The listing builds one solid part. Answer for the finished solid, in the listing's coordinates (mm). A direction names the side the tool comes from. Round coordinates to 2 decimals unless told otherwise and drop trailing zeros. Write each loop counter-clockwise with the first axis right and the second up, starting at its lowest first coordinate (ties: lowest second). Pieces come first, ordered by that corner, then holes. Notation, with made-up numbers: (80.25, 67) - (91.25, 67) arc R13 cw to (91.25, 86) - close; hole circle Ø10 at (-7, 77.25). An arc over 180 degrees is marked (long way). Answer as CSV lines item,"result". Start each with the question number.
Item 1: Which of the six approach directions +Z, -Z, +X, -X, +Y, -Y give full straight-line access (tool end or side, diameter ignored) to faces 5 (the flat face through (30.88, 0, -8)), 6 (the flat face through (-21, 0, 0)), 7 (the flat face through (-5.82, -20.4, -12.2))?
Item 2: Straight lines are drawn through the part: line 1 along Y through (x, z) = (5.75, -50); line 2 along Y through (x, z) = (-4.5, -48.5); line 3 along X through (y, z) = (22.5, -1.5). For each, find the intervals that lie inside material, in ascending order. Write a range as [from, to].
Item 3: A cutting plane is placed at D-D on y = -2. Determine the outline of the cut face in (x, z).
Item 4: A cutting plane is placed at B-B on z = -50. Determine the outline of the cut face in (x, y), and give its area (3 significant figures).
Item 5: A cutting plane is placed at C-C on x = -3. Determine the outline of the cut face in (y, z), and give its area (3 significant figures).
Item 6: Flat-ended cylindrical pins translate along their axes: pin 1 (3 mm diameter, centred on y = 12.5, z = -37.5, fed in from +X); pin 2 (8 mm diameter, centred on y = 18, z = -19.5, fed in from -X); pin 3 (1.5 mm diameter, centred on x = 3, y = -20, fed in from -Z); pin 4 (8 mm diameter, centred on y = -18.5, z = -12, fed in from +X). Find the tip coordinate at first contact, or state that the pin passes through.
Item 7: A cutting plane is placed at A-A on y = 18.2. Determine the outline of the cut face in (x, z), and give its area (3 significant figures).
Item 8: For a pull along X with two mould halves and no side action, classify faces 1 (the cylindrical face through (-8.385, -18.079, -52.747)), 2 (the cylindrical face through (25.28, -25.43, -12.47)), 3 (the cylindrical face through (-20.612, 25.647, 1.528)), 4 (the flat face through (15, 0, -40)) as pulls with the +X half, pulls with the -X half, needs draft (parallel to the pull), parting line crosses it, or undercut.
```python
from build123d import *

# Parameters (mm, degrees)
SKETCH1_W                       = 61.76
SKETCH1_H                       = 56.4
BOSS_EXTRUDE1_DEPTH             = 4
M5X0_8_TAPPED_HOLE1_D           = 4.2
M5X0_8_TAPPED_HOLE1_CSINK_D     = 6
M5X0_8_TAPPED_HOLE1_CSINK_ANGLE = 90
SKETCH37_W                      = 41.76
SKETCH37_H                      = 56.4
SKETCH37_R                      = 2.1
BOSS_EXTRUDE7_DEPTH             = 60
CUT_EXTRUDE2_DEPTH              = 57.4
CBORE_FOR_M5_SHCS3_D            = 5.5
CBORE_FOR_M5_SHCS3_CBORE_D      = 10
CBORE_FOR_M5_SHCS3_CBORE_DEPTH  = 36.7
CHAMFER7_SIZE                   = 0.5


with BuildPart() as part:
    # Sketch1 → Boss-Extrude1 (new body)
    with BuildSketch(Plane.XY):
        Rectangle(SKETCH1_W, SKETCH1_H)
    extrude(amount=BOSS_EXTRUDE1_DEPTH)

    # M5x0.8 Tapped Hole1 (through all)
    with Locations(Plane.XY.offset(4)):
        with Locations((26.245, 23.565), (26.245, -23.565), (-20.885, -23.565), (-20.885, 23.565)):
            CounterSinkHole(M5X0_8_TAPPED_HOLE1_D / 2, M5X0_8_TAPPED_HOLE1_CSINK_D / 2, counter_sink_angle=M5X0_8_TAPPED_HOLE1_CSINK_ANGLE)

    # Sketch37 → Boss-Extrude7 (add)
    with BuildSketch(Plane(origin=(0, 0, 0), x_dir=(-1, 0, 0), z_dir=(0, 0, -1))):
        with Locations((-10, 0)):
            Rectangle(SKETCH37_W, SKETCH37_H)
        with Locations((-26.245, 23.565)):
            Circle(SKETCH37_R, mode=Mode.SUBTRACT)
        with Locations((-26.245, -23.565)):
            Circle(SKETCH37_R, mode=Mode.SUBTRACT)
    extrude(amount=BOSS_EXTRUDE7_DEPTH)

    # Sketch40 → Cut-Extrude2 (cut, through all)
    with BuildSketch(Plane.XZ.offset(28.2)):
        Polygon((-0.88, -60), (30.88, -20), (30.88, -60), align=None)
    extrude(amount=-CUT_EXTRUDE2_DEPTH, mode=Mode.SUBTRACT)

    # CBORE for M5 SHCS3 (through all)
    with Locations(Plane(origin=(30.88, 0, 0), x_dir=(0, 0, -1), z_dir=(1, 0, 0))):
        with Locations((10, -18.2), (10, 18.2), (50, 18.2), (50, -18.2)):
            CounterBoreHole(CBORE_FOR_M5_SHCS3_D / 2, CBORE_FOR_M5_SHCS3_CBORE_D / 2, CBORE_FOR_M5_SHCS3_CBORE_DEPTH)

    # Chamfer7
    chamfer7_edges = [part.edges().sort_by_distance(p)[0] for p in [
        (0, -28.2, 4),
        (-20.88, 28.2, 0),
        (-5.88, 28.2, -60),
        (-10.88, -28.2, -30),
        (-10.88, 28.2, -30),
        (-20.88, -28.2, 0),
        (-5.88, -28.2, -60),
        (15, 28.2, -40),
        (15, -28.2, -40),
        (30.88, -28.2, -8),
        (-30.88, -28.2, 2),
        (-30.88, 28.2, 2),
        (30.88, 28.2, -8),
        (0, 28.2, 4),
    ]]
    chamfer(chamfer7_edges, length=CHAMFER7_SIZE)


solid = part.part
```
Geometry says:
1,face 5,"+Z, -Z, +X, +Y, -Y"
1,face 6,"-Z, -X, +Y, -Y"
1,face 7,"+X"
2,line 1,"y = [-28.2, -23.2], [-13.2, 13.2], [23.2, 28.2]"
2,line 2,"y = [-28.2, -22.97], [-13.43, 13.43], [22.97, 28.2]"
2,line 3,"x = [-10.88, 24.44], [28.05, 30.88]"
3,outline,"(-30.88, 0) - (-10.88, 0) - (-10.88, -60) - (-0.88, -60) - (30.88, -20) - (30.88, 4) - (-30.88, 4) - close"
4,outline,"(-10.88, -27.7) - (-10.38, -28.2) - (6.42, -28.2) - (7.06, -27.7) - (7.06, -23.2) - (-5.82, -23.2) - (-5.82, -20.95) - (-10.88, -20.95) - close; (-10.88, -15.45) - (-5.82, -15.45) - (-5.82, -13.2) - (7.06, -13.2) - (7.06, 13.2) - (-5.82, 13.2) - (-5.82, 15.45) - (-10.88, 15.45) - close; (-10.88, 20.95) - (-5.82, 20.95) - (-5.82, 23.2) - (7.06, 23.2) - (7.06, 27.7) - (6.42, 28.2) - (-10.38, 28.2) - (-10.88, 27.7) - close"
4,area,"698 mm^2"
5,outline,"(-28.2, -59.5) - (-27.7, -60) - (27.7, -60) - (28.2, -59.5) - (28.2, 3.5) - (27.7, 4) - (-27.7, 4) - (-28.2, 3.5) - close; hole circle Ø10 at (-18.2, -50); hole circle Ø10 at (-18.2, -10); hole circle Ø10 at (18.2, -50); hole circle Ø10 at (18.2, -10)"
5,area,"3,290 mm^2"
6,pin 1,"stops at x = 18.18"
6,pin 2,"stops at x = -10.88"
6,pin 3,"stops at z = -56.06"
6,pin 4,"stops at x = 30.88"
7,outline,"(-30.88, 0) - (-10.88, 0) - (-10.88, -7.25) - (-5.82, -7.25) - (-5.82, -5) - (30.88, -5) - (30.88, 4) - (-30.88, 4) - close; (-10.88, -60) - (-0.88, -60) - (3.09, -55) - (-5.82, -55) - (-5.82, -52.75) - (-10.88, -52.75) - close; (-10.88, -47.25) - (-5.82, -47.25) - (-5.82, -45) - (11.03, -45) - (30.88, -20) - (30.88, -15) - (-5.82, -15) - (-5.82, -12.75) - (-10.88, -12.75) - close"
7,area,"1,570 mm^2"
8,face 1,"needs draft"
8,face 2,"undercut"
8,face 3,"undercut"
8,face 4,"pulls with the +X half"
